Verification items for the finished model (mm, model axes). A direction names the side the tool comes from. Coordinates: 2 decimals unless noted, no trailing zeros. Order: outer loops, then holes, each group sorted by start corner. A loop starts at its lowest first (then second) coordinate and runs counter-clockwise, first axis right, second up. Notation, with made-up numbers: M 12.5,49.5 L 38.5,49.5 A18 cw 38.5,59.5 Z; hole C 23.25,61 d5. An arc over 180 degrees is marked long. Write item = value, one per line.
```python
from build123d import *

# Parameters (mm, degrees)
BRIDA_BASE1_DEPTH           = 75
CORTAR_EXTRUIR1_START       = -9.525
CORTAR_EXTRUIR1_OUTLINE_W   = 49.6
CORTAR_EXTRUIR1_OUTLINE_H   = 121
CORTAR_EXTRUIR1_DEPTH       = 9.525
CORTAR_EXTRUIR1_START_2     = -53.5025
CORTAR_EXTRUIR1_2_OUTLINE_W = 49.6
CORTAR_EXTRUIR1_2_OUTLINE_H = 94.7625
CORTAR_EXTRUIR1_2_DEPTH     = 43.9775
CORTAR_EXTRUIR2_DEPTH       = 10
CORTAR_EXTRUIR3_DEPTH       = 10


# Read off the part's stored shape, not the designer's step: Cortar-Extruir1
# Sheet-metal steps are written as plain solids
with BuildPart() as part:
    # Croquis1 → Brida base1 (new, symmetric)
    with BuildSketch(Plane.XY):
        with BuildLine():
            Line((33.76, 105), (33.76, 19.7625))
            ThreePointArc((33.76, 19.7625), (35.154903955, 16.394903955), (38.5225, 15))
            Line((38.5225, 15), (72.975, 15))
            ThreePointArc((72.975, 15), (79.710192091, 12.210192091), (82.5, 5.475))
            Line((82.5, 5.475), (82.5, -95.475))
            ThreePointArc((82.5, -95.475), (79.710192091, -102.210192091), (72.975, -105))
            Line((72.975, -105), (-82.5, -105))
            Line((-82.5, -105), (-82.5, -100.2375))
            Line((-82.5, -100.2375), (72.975, -100.2375))
            ThreePointArc((72.975, -100.2375), (76.342596045, -98.842596045), (77.7375, -95.475))
            Line((77.7375, -95.475), (77.7375, 5.475))
            ThreePointArc((77.7375, 5.475), (76.342596045, 8.842596045), (72.975, 10.2375))
            Line((72.975, 10.2375), (38.5225, 10.2375))
            ThreePointArc((38.5225, 10.2375), (31.787307909, 13.027307909), (28.9975, 19.7625))
            Line((28.9975, 19.7625), (28.9975, 105))
            Line((28.9975, 105), (33.76, 105))
        make_face()
    extrude(amount=BRIDA_BASE1_DEPTH, both=True)

    # Cortar-Extruir1 outline → Cortar-Extruir1 (cut)
    with BuildSketch(Plane(origin=(82.5, 0, 0), x_dir=(0, 0, -1), z_dir=(1, 0, 0)).offset(CORTAR_EXTRUIR1_START)):
        with Locations((50.2, -45.5)):
            Rectangle(CORTAR_EXTRUIR1_OUTLINE_W, CORTAR_EXTRUIR1_OUTLINE_H)
        with Locations((-50.2, -45.5)):
            Rectangle(CORTAR_EXTRUIR1_OUTLINE_W, CORTAR_EXTRUIR1_OUTLINE_H)
    extrude(amount=CORTAR_EXTRUIR1_DEPTH, mode=Mode.SUBTRACT)

    # Cortar-Extruir1 2 outline → Cortar-Extruir1 2 (cut)
    with BuildSketch(Plane(origin=(82.5, 0, 0), x_dir=(0, 0, -1), z_dir=(1, 0, 0)).offset(CORTAR_EXTRUIR1_START_2)):
        with Locations((50.2, 57.61875)):
            Rectangle(CORTAR_EXTRUIR1_2_OUTLINE_W, CORTAR_EXTRUIR1_2_OUTLINE_H)
        with Locations((-50.2, 57.61875)):
            Rectangle(CORTAR_EXTRUIR1_2_OUTLINE_W, CORTAR_EXTRUIR1_2_OUTLINE_H)
    extrude(amount=CORTAR_EXTRUIR1_2_DEPTH, mode=Mode.SUBTRACT)

    # Croquis7 → Cortar-Extruir2 (cut)
    with BuildSketch(Plane(origin=(33.76, 0, 0), x_dir=(0, 0, -1), z_dir=(1, 0, 0))):
        with BuildLine():
            Line((-15, 42.5), (-15, 67.5))
            ThreePointArc((-15, 67.5), (-12.5, 65), (-10, 67.5))
            Line((-10, 67.5), (-10, 42.5))
            ThreePointArc((-10, 42.5), (-12.5, 40), (-15, 42.5))
        make_face()
        with BuildLine():
            ThreePointArc((-15, 67.5), (-12.5, 65), (-10, 67.5))
            ThreePointArc((-10, 67.5), (-12.5, 70), (-15, 67.5))
        make_face()
        with BuildLine():
            ThreePointArc((-10, 67.5), (-12.5, 70), (-15, 67.5))
            Line((-15, 67.5), (-15, 92.5))
            ThreePointArc((-15, 92.5), (-12.5, 95), (-10, 92.5))
            Line((-10, 92.5), (-10, 67.5))
        make_face()
        with BuildLine():
            ThreePointArc((15, 67.5), (12.5, 70), (10, 67.5))
            Line((10, 67.5), (10, 92.5))
            ThreePointArc((10, 92.5), (12.5, 95), (15, 92.5))
            Line((15, 92.5), (15, 67.5))
        make_face()
        with BuildLine():
            ThreePointArc((10, 67.5), (12.5, 65), (15, 67.5))
            ThreePointArc((15, 67.5), (12.5, 70), (10, 67.5))
        make_face()
        with BuildLine():
            Line((10, 42.5), (10, 67.5))
            ThreePointArc((10, 67.5), (12.5, 65), (15, 67.5))
            Line((15, 67.5), (15, 42.5))
            ThreePointArc((15, 42.5), (12.5, 40), (10, 42.5))
        make_face()
    extrude(amount=-CORTAR_EXTRUIR2_DEPTH, mode=Mode.SUBTRACT)

    # Croquis8 → Cortar-Extruir3 (cut)
    with BuildSketch(Plane.XZ.offset(105)):
        with BuildLine():
            Line((-72.5, -60), (-72.5, 60))
            ThreePointArc((-72.5, 60), (-68.3, 64.2), (-64.1, 60))
            Line((-64.1, 60), (-64.1, -60))
            ThreePointArc((-64.1, -60), (-68.3, -64.2), (-72.5, -60))
        make_face()
        with BuildLine():
            Line((-12.5, -60), (-12.5, 60))
            ThreePointArc((-12.5, 60), (-8.3, 64.2), (-4.1, 60))
            Line((-4.1, 60), (-4.1, -60))
            ThreePointArc((-4.1, -60), (-8.3, -64.2), (-12.5, -60))
        make_face()
        with BuildLine():
            Line((47.5, -60), (47.5, 60))
            ThreePointArc((47.5, 60), (51.7, 64.2), (55.9, 60))
            Line((55.9, 60), (55.9, -60))
            ThreePointArc((55.9, -60), (51.7, -64.2), (47.5, -60))
        make_face()
        with BuildLine():
            Line((-68.3, 4.2), (51.7, 4.2))
            ThreePointArc((51.7, 4.2), (55.9, 0), (51.7, -4.2))
            Line((51.7, -4.2), (-68.3, -4.2))
            ThreePointArc((-68.3, -4.2), (-72.5, 0), (-68.3, 4.2))
        make_face()
    extrude(amount=-CORTAR_EXTRUIR3_DEPTH, mode=Mode.SUBTRACT)


solid = part.part
```
Item 1: Sectioned sample at A-A, the plane z = 21.5. Give the number of separate pieces and of enclosed holes in the cut face, then the cut area to 3 significant figures.
Report:
separate_pieces = 4
enclosed_holes = 0
area = 1,830 mm^2
Item 2: Gauge pin test, flat ends, axial feed: pin 1 (5 mm diameter, centred on x = 30.5, y = 78, fed in from -Z); pin 2 (2.5 mm diameter, centred on y = -102, z = 44, fed in from +X) (3 decimals); pin 3 (4 mm diameter, centred on y = 45.5, z = -4.5, fed in from -X). Record the tip position at first contact, or that the pin passes through.
Report:
pin_1 = -25.4
pin_2 = 72.975
pin_3 = 29
Item 3: Tool access check on faces 3 (the cylindrical face through (76.379, 8.805, 0.356)), 4 (the flat face through (72.975, -103, 51)), 5 (the flat face through (-64.1, -103, -32)). Record the directions out of +Z, -Z, +X, -X, +Y, -Y that give a thin tool (end or side, any length) a straight path to the whole face; none if there is none.
Report:
face_3 = +Z, -Z, -X
face_4 = +Z, +X, +Y, -Y
face_5 = +Y, -Y
Item 4: Sectioned sample at D-D, the plane z = 42.5. Enter the section's corners in (x, y) (1 decimal).
Report:
outline = M -82.5,-105 L -72.5,-105 L -72.5,-100.2 L -82.5,-100.2 Z; M -64.1,-105 L -12.5,-105 L -12.5,-100.2 L -64.1,-100.2 Z; M -4.1,-105 L 47.5,-105 L 47.5,-100.2 L -4.1,-100.2 Z; M 55.9,-105 L 73,-105 L 73,-100.2 L 55.9,-100.2 Z
Item 5: Sectioned sample at B-B, the plane y = 75. Enter the section's corners in (x, z), then the cut area to 3 significant figures.
Report:
outline = M 29,-25.4 L 33.76,-25.4 L 33.76,-15 L 29,-15 Z; M 29,-10 L 33.76,-10 L 33.76,10 L 29,10 Z; M 29,15 L 33.76,15 L 33.76,25.4 L 29,25.4 Z
area = 194 mm^2
Item 6: Sectioned sample at C-C, the plane x = 64. Enter the section's corners in (y, z).
Report:
outline = M -105,-75 L -100.24,-75 L -100.24,75 L -105,75 Z; M 10.24,-25.4 L 15,-25.4 L 15,25.4 L 10.24,25.4 Z
Item 7: Scan lines: L1, parallel to Y at x = 61, z = 13; L2, parallel to Y at x = -43.5, z = -34; L3, parallel to X at y = 26.5, z = -4. Record each from-to range of solid material in increasing order. Write a range as from..to.
Report:
L1 = -105..-100.24, 10.24..15
L2 = -105..-100.24
L3 = 29..33.76
Item 8: Release check for a two-part mould opening along Y. For faces 1 (the flat face through (-12.5, -103, 32)), 2 (the flat face through (31, 67, -15)) record: pulls with the +Y half, pulls with the -Y half, needs draft (parallel to the pull), parting line crosses it, or undercut.
Report:
face_1 = needs draft
face_2 = undercut
